from build123d import *

# Parameters (mm, degrees)
SKETCH1_W           = 77.2
SKETCH1_H           = 114.3
BOSS_EXTRUDE1_DEPTH = 77.2
SKETCH2_W           = 70.58
SKETCH2_H           = 70.58
CUT_EXTRUDE1_DEPTH  = 107.95
SKETCH3_R           = 10.5
SKETCH3_R_2         = 1.7
CUT_EXTRUDE2_DEPTH  = 115.3
SKETCH4_R           = 73.025
SKETCH4_R_2         = 1.7
SKETCH4_R_3         = 10.5
BOSS_EXTRUDE4_DEPTH = 6.35


with BuildPart() as part:
    # Sketch1 → Boss-Extrude1 (new body)
    with BuildSketch(Plane.XY):
        with Locations((38.6, 57.15)):
            Rectangle(SKETCH1_W, SKETCH1_H)
    extrude(amount=-BOSS_EXTRUDE1_DEPTH)

    # Sketch2 → Cut-Extrude1 (cut)
    with BuildSketch(Plane.XZ):
        with Locations((38.6, -38.6)):
            Rectangle(SKETCH2_W, SKETCH2_H)
    extrude(amount=-CUT_EXTRUDE1_DEPTH, mode=Mode.SUBTRACT)

    # Sketch3 → Cut-Extrude2 (cut, through all)
    with BuildSketch(Plane(origin=(0, 114.3, 0), x_dir=(1, 0, 0), z_dir=(0, 1, 0))):
        with Locations((38.6, 38.6)):
            Circle(SKETCH3_R)
        with Locations((38.6, 55.1)):
            Circle(SKETCH3_R_2)
        with Locations((55.1, 38.6)):
            Circle(SKETCH3_R_2)
        with Locations((38.6, 22.1)):
            Circle(SKETCH3_R_2)
        with Locations((22.1, 38.6)):
            Circle(SKETCH3_R_2)
    extrude(amount=-CUT_EXTRUDE2_DEPTH, mode=Mode.SUBTRACT)

    # Sketch4 → Boss-Extrude4 (add)
    with BuildSketch(Plane(origin=(0, 114.3, 0), x_dir=(1, 0, 0), z_dir=(0, 1, 0))):
        with Locations((38.6, 38.6)):
            Circle(SKETCH4_R)
        with Locations((38.6, 55.1)):
            Circle(SKETCH4_R_2, mode=Mode.SUBTRACT)
        with Locations((55.1, 38.6)):
            Circle(SKETCH4_R_2, mode=Mode.SUBTRACT)
        with Locations((38.6, 22.1)):
            Circle(SKETCH4_R_2, mode=Mode.SUBTRACT)
        with Locations((22.1, 38.6)):
            Circle(SKETCH4_R_2, mode=Mode.SUBTRACT)
        with Locations((38.6, 38.6)):
            Circle(SKETCH4_R_3, mode=Mode.SUBTRACT)
    extrude(amount=-BOSS_EXTRUDE4_DEPTH)


solid = part.part
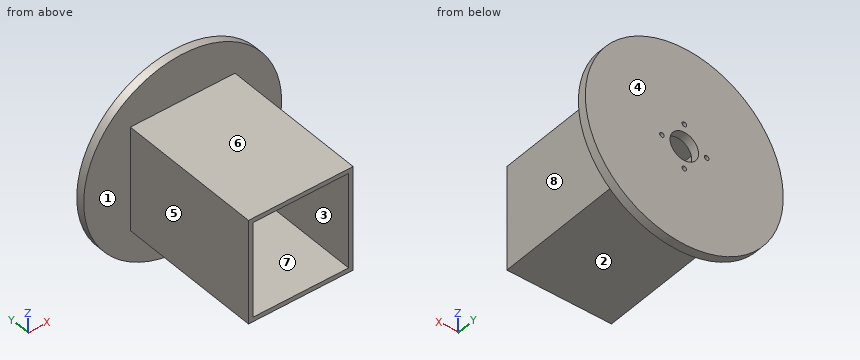
Input: part model. Units: mm. Frame: model coordinates. Face numbers are marked on the shaded views. A direction names the side the tool comes from. Give positions to 0.01 mm unless a question says otherwise; leave off trailing zeros. Order: outer loops, then holes, each group sorted by start corner. A loop starts at its lowest first (then second) coordinate and runs counter-clockwise, first axis right, second up. Notation, with made-up numbers: (33, -15) -> (83, -15) arc R7 cw to (83, -9) -> close; hole circle Ø4 at (71, -16.5). An arc over 180 degrees is marked (long way). Use one line per item in the form item = value.
1) Section A-A, the plane x = 46. Return loops of the section in (y, z), and give its area (3 significant figures).
Response values:
outline = (0, -77.2) -> (107.95, -77.2) -> (107.95, -111.25) -> (114.3, -111.25) -> (114.3, -46.05) -> (107.95, -46.05) -> (107.95, -73.89) -> (0, -73.89) -> close; (0, -3.31) -> (107.95, -3.31) -> (107.95, -31.15) -> (114.3, -31.15) -> (114.3, 34.05) -> (107.95, 34.05) -> (107.95, 0) -> (0, 0) -> close
area = 1,540 mm^2
2) Reachability of the marked faces 4, 5, 6, 7 and 8 from +Z, -Z, +X, -X, +Y, -Y: full face, straight path, thin tool, end or side. Return the list, or none.
Response values:
face_4 = +Z, -Z, +X, -X, +Y
face_5 = +Z, -Z, -X, -Y
face_6 = +Z, +X, -X, -Y
face_7 = -Y
face_8 = +Z, -Z, +X, -Y
3) Mould query, pull axis Z, two halves, no side actions, for the marked faces 1, 2 and 3. Classes: pulls with the +Z half, pulls with the -Z half, needs draft (parallel to the pull), parting line crosses it, or undercut.
Response values:
face_1 = needs draft
face_2 = pulls with the -Z half
face_3 = undercut
4) Line query: probe 1 along X at (y, z) = (109.75, -38.6) (3 decimals); probe 2 along X at (y, z) = (45, -17); probe 3 along X at (y, z) = (110, -38). Output: solid intervals per line, ascending.
Response values:
probe_1 = -34.425 to 20.4, 23.8 to 28.1, 49.1 to 53.4, 56.8 to 111.625
probe_2 = 0 to 3.31, 73.89 to 77.2
probe_3 = -34.42 to 20.51, 23.69 to 28.12, 49.08 to 53.51, 56.69 to 111.62
5) Section D-D, the plane x = 95.5. Return loops of the section in (y, z), and give its area (3 significant figures).
Response values:
outline = (107.95, -84.37) -> (114.3, -84.37) -> (114.3, 7.17) -> (107.95, 7.17) -> close
area = 581 mm^2
6) Section B-B, the plane y = 73.5. Return loops of the section in (x, z).
Response values:
outline = (0, -77.2) -> (77.2, -77.2) -> (77.2, 0) -> (0, 0) -> close; hole (3.31, -73.89) -> (73.89, -73.89) -> (73.89, -3.31) -> (3.31, -3.31) -> close
7) First-contact query: pin 1 Ø8 at (y, z) = (55.5, -71) entering from -X; pin 2 Ø4.5 at (x, z) = (22.1, -38.6) entering from -Y; pin 3 Ø23 at (x, y) = (34, 78.5) entering from +Z. Flat tips, straight axial feed; report the tip coordinate or a pass-through.
Response values:
pin_1 = 0
pin_2 = 107.95
pin_3 = 0
8) Section C-C, the plane z = -95.5. Return loops of the section in (x, y), and give its area (3 significant figures).
Response values:
outline = (-7.17, 107.95) -> (84.37, 107.95) -> (84.37, 114.3) -> (-7.17, 114.3) -> close
area = 581 mm^2
